```python
from build123d import *

# Parameters (mm, degrees)
BOSS_EXTRUDE1_DEPTH = 2.276130482


with BuildPart() as part:
    # Sketch1 → Boss-Extrude1 (new body)
    with BuildSketch(Plane.XY):
        with BuildLine():
            ThreePointArc((-7.498149452, 0), (0, 7.498149452), (7.498149452, 0))
            Line((7.498149452, 0), (25.4, 0))
            ThreePointArc((25.4, 0), (0, 25.4), (-25.4, 0))
            Line((-25.4, 0), (-7.498149452, 0))
        make_face()
        with BuildLine():
            Line((25.4, 0), (7.498149452, 0))
            ThreePointArc((7.498149452, 0), (0, -7.498149452), (-7.498149452, 0))
            Line((-7.498149452, 0), (-25.4, 0))
            ThreePointArc((-25.4, 0), (-17.960512225, -17.960512259), (4.9e-08, -25.4))
            ThreePointArc((4.9e-08, -25.4), (17.960512259, -17.960512225), (25.4, 0))
        make_face()
        with BuildLine():
            Line((25.4, -50.8), (25.4, 0))
            ThreePointArc((25.4, 0), (17.960512259, -17.960512225), (4.9e-08, -25.4))
            ThreePointArc((4.9e-08, -25.4), (17.960512259, -32.839487775), (25.4, -50.8))
        make_face()
        with BuildLine():
            ThreePointArc((4.9e-08, -25.4), (-17.960512225, -17.960512259), (-25.4, 0))
            Line((-25.4, 0), (-25.4, -50.8))
            ThreePointArc((-25.4, -50.8), (-17.960512225, -32.839487741), (4.9e-08, -25.4))
        make_face()
        with BuildLine():
            ThreePointArc((-25.4, -50.8), (0, -76.2), (25.4, -50.8))
            Line((25.4, -50.8), (12.7, -50.8))
            ThreePointArc((12.7, -50.8), (0, -63.5), (-12.7, -50.8))
            Line((-12.7, -50.8), (-25.4, -50.8))
        make_face()
        with BuildLine():
            Line((12.7, -50.8), (25.4, -50.8))
            ThreePointArc((25.4, -50.8), (17.960512259, -32.839487775), (4.9e-08, -25.4))
            ThreePointArc((4.9e-08, -25.4), (-17.960512225, -32.839487741), (-25.4, -50.8))
            Line((-25.4, -50.8), (-12.7, -50.8))
            ThreePointArc((-12.7, -50.8), (0, -38.1), (12.7, -50.8))
        make_face()
    extrude(amount=BOSS_EXTRUDE1_DEPTH)


solid = part.part
```
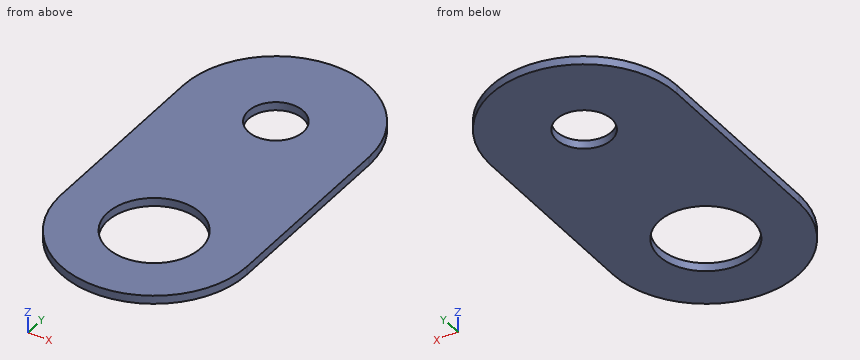
Could you check a few things on this model? Use its own coordinates, in mm. Coordinates: 2 decimals unless noted, no trailing zeros. Order: outer loops, then holes, each group sorted by start corner. A loop starts at its lowest first (then second) coordinate and runs counter-clockwise, first axis right, second up. Notation, with made-up numbers: M 11,25.25 L 17,25.25 A8 cw 17,39.25 Z; hole C 34.25,74.5 d11. An arc over 180 degrees is marked long. Use a Markdown table: item, result. Add a question column.
Q1. I want a section at C-C on z = 0.6. List the corners of the cut face in (x, y) for me.
Q2. I want a section at D-D on x = -9. List the corners of the cut face in (y, z) for me.
Q3. If I drill on L1, parallel to Y at x = 0, z = 0.6; L2, parallel to X at y = -58.5, z = 0.3; L3, parallel to Y at x = -10, z = 0.75, over which ranges is the centre line in solid material (lowest first)?
Q4. I want a section at A-A on x = 0. List the corners of the cut face in (y, z) for me, then the cut area to 3 significant figures.
Q5. I want a section at B-B on y = -48.5. List the corners of the cut face in (x, z) for me.
Checked values:
| question | item | result |
|---|---|---|
| 1 | outline | M -25.4,-50.8 A25.4 ccw 25.4,-50.8 L 25.4,0 A25.4 ccw -25.4,0 Z; hole C 0,-50.8 d25.4; hole C 0,0 d15 |
| 2 | outline | M -74.55,0 L -59.76,0 L -59.76,2.28 L -74.55,2.28 Z; M -41.84,0 L 23.75,0 L 23.75,2.28 L -41.84,2.28 Z |
| 3 | L1 | -76.2 to -63.5, -38.1 to -7.5, 7.5 to 25.4 |
| 3 | L2 | -24.2 to -10.1, 10.1 to 24.2 |
| 3 | L3 | -74.15 to -58.63, -42.97 to 23.35 |
| 4 | outline | M -76.2,0 L -63.5,0 L -63.5,2.28 L -76.2,2.28 Z; M -38.1,0 L -7.5,0 L -7.5,2.28 L -38.1,2.28 Z; M 7.5,0 L 25.4,0 L 25.4,2.28 L 7.5,2.28 Z |
| 4 | area | 139 mm² |
| 5 | outline | M -25.4,0 L -12.49,0 L -12.49,2.28 L -25.4,2.28 Z; M 12.49,0 L 25.4,0 L 25.4,2.28 L 12.49,2.28 Z |
